Can you work these out from the drawing? Everything is in mm from the part's minimum corner. A direction names the side the tool comes from. Coordinates: 2 decimals unless noted, no trailing zeros. Write each loop counter-clockwise with the first axis right and the second up, starting at its lowest first coordinate (ties: lowest second). Pieces come first, ordered by that corner, then holes. Notation, with made-up numbers: (30, 38) -> (74, 38) arc R14 ccw to (74, 50) -> close; hole circle Ø8 at (37, 28). An arc over 180 degrees is marked (long way). Use a Markdown table: item, result. Add a question column.
Item 1: Imagine slicing it at C-C, the plane x = 6.35. Write out the boundary of the cut face in (y, z) (1 decimal), and give its area (3 significant figures).
Item 2: Imagine slicing it at D-D, the plane y = 3. Write out the boundary of the cut face in (x, z), and give its area (3 significant figures).
Item 3: Imagine slicing it at B-B, the plane z = 19.05. Write out the boundary of the cut face in (x, y) (1 decimal).
Item 4: Will these pins go through, and if not, where does the flat tip stop? pin 1 Ø3.5 at (y, z) = (2.5, 4.5) entering from +X; pin 2 Ø6 at (x, z) = (8.5, 4.5) entering from -Y; pin 3 Ø3 at (y, z) = (8.5, 9) entering from -X.
Item 5: Imagine slicing it at A-A, the plane z = 3.75. Write out the boundary of the cut face in (x, y).
Item 6: On a 3-axis mill with a long thin cutter (end or side, diameter ignored), from which of +Z, -Z, +X, -X, +Y, -Y can I reach the whole of each face in a straight line? I mean the marked faces 5, 6, 7, 8 and 9. Say none if no direction works.
Item 7: If we mould it in two halves opening along Y, with no side actions, what happens to the marked faces 1, 2, 3 and 4? For each: pulls with the +Y half, pulls with the -Y half, needs draft (parallel to the pull), parting line crosses it, or undercut.
Item 8: If I drill on line 1 along Y through (x, z) = (2.75, 2.5); line 2 along Z through (x, y) = (11.5, 6); line 3 along X through (y, z) = (2.5, 8.75), over which ranges is the centre line in solid material (lowest first)? Write a range as from..to.
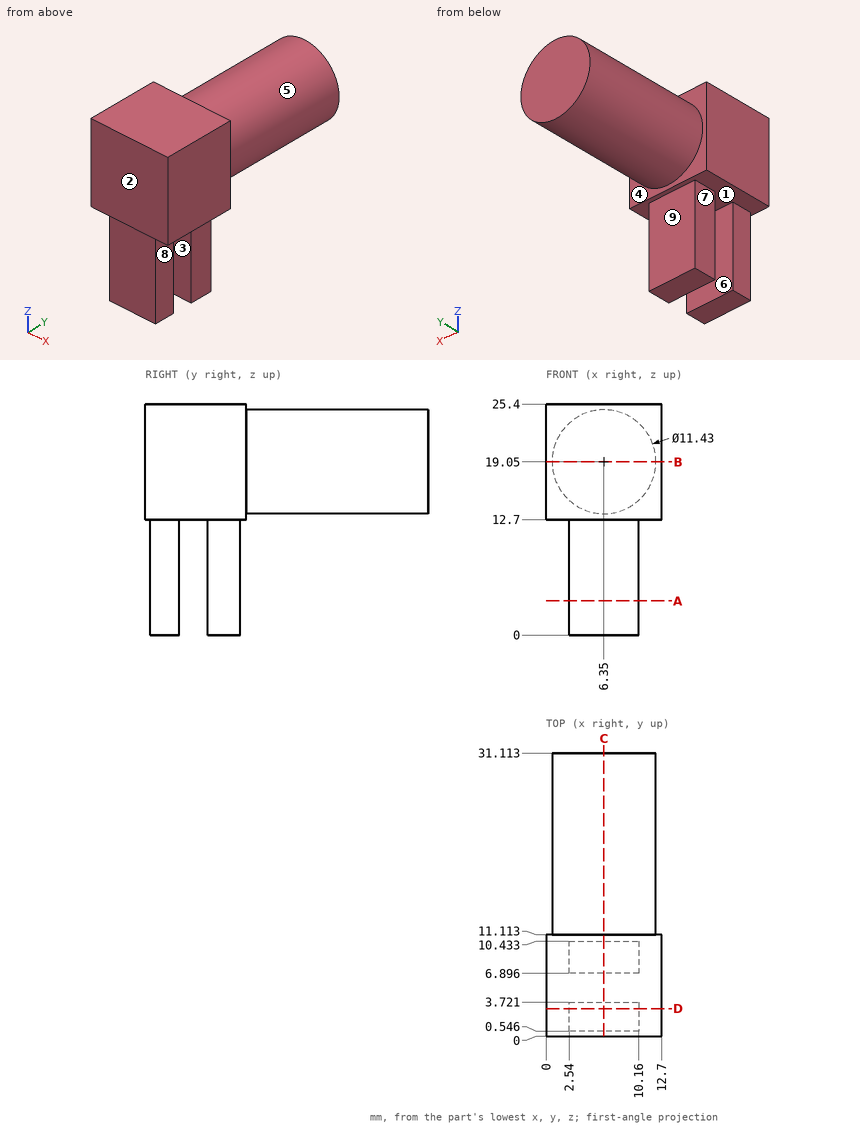
Ans:
| question | item | result |
|---|---|---|
| 1 | outline | (0, 12.7) -> (0.5, 12.7) -> (0.5, 0) -> (3.7, 0) -> (3.7, 12.7) -> (6.9, 12.7) -> (6.9, 0) -> (10.4, 0) -> (10.4, 12.7) -> (11.1, 12.7) -> (11.1, 13.3) -> (31.1, 13.3) -> (31.1, 24.8) -> (11.1, 24.8) -> (11.1, 25.4) -> (0, 25.4) -> close |
| 1 | area | 455 mm^2 |
| 2 | outline | (0, 12.7) -> (2.54, 12.7) -> (2.54, 0) -> (10.16, 0) -> (10.16, 12.7) -> (12.7, 12.7) -> (12.7, 25.4) -> (0, 25.4) -> close |
| 2 | area | 258 mm^2 |
| 3 | outline | (0, 0) -> (12.7, 0) -> (12.7, 11.1) -> (12.1, 11.1) -> (12.1, 31.1) -> (0.6, 31.1) -> (0.6, 11.1) -> (0, 11.1) -> close |
| 4 | pin 1 | stops at x = 10.16 |
| 4 | pin 2 | stops at y = 0.55 |
| 4 | pin 3 | stops at x = 2.54 |
| 5 | outline | (2.54, 0.55) -> (10.16, 0.55) -> (10.16, 3.72) -> (2.54, 3.72) -> close; (2.54, 6.9) -> (10.16, 6.9) -> (10.16, 10.43) -> (2.54, 10.43) -> close |
| 6 | face 5 | +Y |
| 6 | face 6 | -Z, +X, -X |
| 6 | face 7 | -Z, -X, +Y, -Y |
| 6 | face 8 | -Z, +X, +Y, -Y |
| 6 | face 9 | -Z, +X, -X, +Y |
| 7 | face 1 | undercut |
| 7 | face 2 | pulls with the -Y half |
| 7 | face 3 | undercut |
| 7 | face 4 | pulls with the +Y half |
| 8 | line 1 | y = 0.55..3.72, 6.9..10.43 |
| 8 | line 2 | z = 12.7..25.4 |
| 8 | line 3 | x = 2.54..10.16 |
